The figure shows three views and two pictorial views of one solid part (mm, origin at its lowest corner). Answer the questions. Give positions to 0.01 mm unless a question says otherwise; leave off trailing zeros. Write each loop counter-clockwise with the first axis right and the second up, starting at its lowest first coordinate (ties: lowest second). Pieces come first, ordered by that corner, then holes. Notation, with made-up numbers: (-33.75, 5) -> (19.25, 5) arc R24 cw to (19.25, 42) -> close; hole circle Ø3 at (58, -6). An arc over 180 degrees is marked (long way). Write item = value, one per line. Start each with the question number.
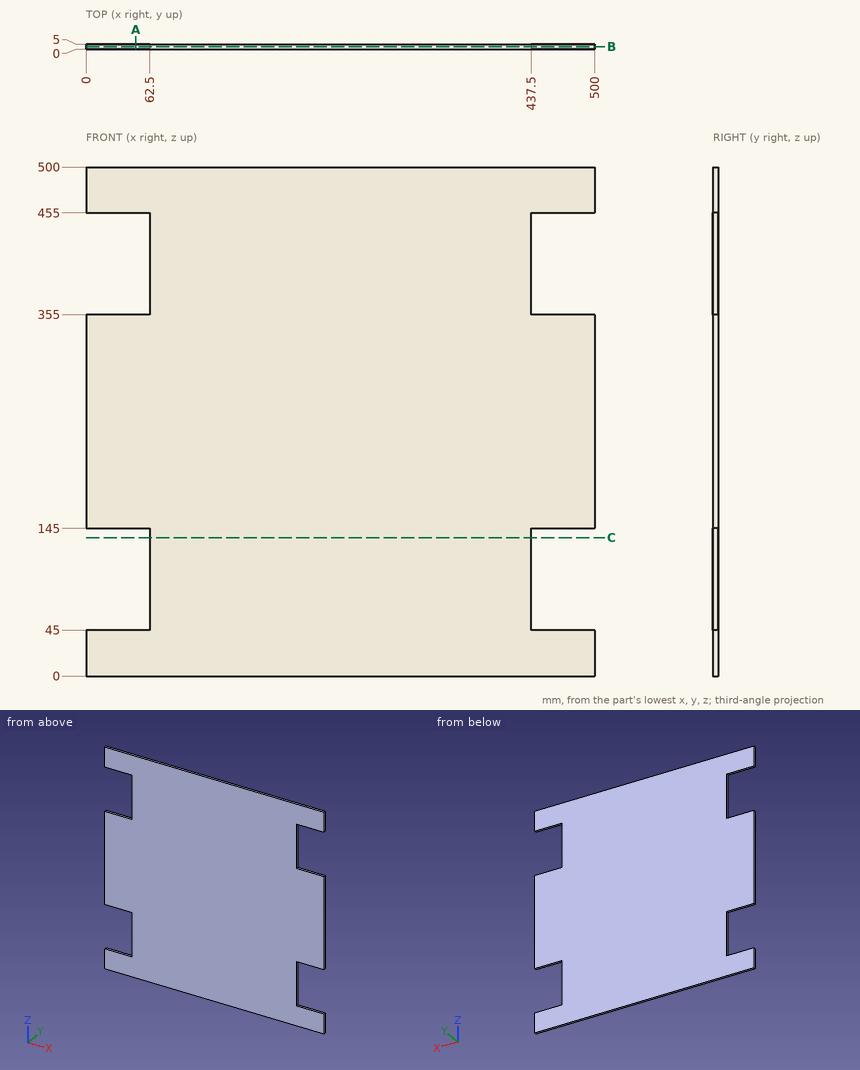
(1) Each of these flat-tipped pins is pushed along its axis until it touches: pin 1 (1.5 mm diameter, centred on x = 332.5, y = 1, fed in from -Z); pin 2 (2.5 mm diameter, centred on y = 3.5, z = 70.5, fed in from +X). Where does it stop, or does it pass through?
(2) A cutting plane is placed at A-A, the plane x = 49. Write down the section's boundary in (y, z).
(3) A cutting plane is placed at C-C, the plane z = 136. Write down the section's boundary in (x, y), then the cut area to 4 significant figures.
(4) Find the intervals of material crossed by line 1 along Z through (x, y) = (22.5, 4.65); line 2 along X through (y, z) = (1.35, 128), in increasing order.
(5) A cutting plane is placed at B-B, the plane y = 2.4. Write down the section's boundary in (x, z).
Results list:
q1.pin_1 = 0
q1.pin_2 = 437.5
q2.outline = (0, 0) -> (5, 0) -> (5, 45) -> (0, 45) -> close; (0, 145) -> (5, 145) -> (5, 355) -> (0, 355) -> close; (0, 455) -> (5, 455) -> (5, 500) -> (0, 500) -> close
q3.outline = (62.5, 0) -> (437.5, 0) -> (437.5, 5) -> (62.5, 5) -> close
q3.area = 1,875 mm²
q4.line_1 = 0 to 45, 145 to 355, 455 to 500
q4.line_2 = 62.5 to 437.5
q5.outline = (0, 0) -> (500, 0) -> (500, 45) -> (437.5, 45) -> (437.5, 145) -> (500, 145) -> (500, 355) -> (437.5, 355) -> (437.5, 455) -> (500, 455) -> (500, 500) -> (0, 500) -> (0, 455) -> (62.5, 455) -> (62.5, 355) -> (0, 355) -> (0, 145) -> (62.5, 145) -> (62.5, 45) -> (0, 45) -> close
